Here's the drawing with two shaded views (mm, measured from the low corner). I have some questions. Round coordinates to 2 decimals unless told otherwise and drop trailing zeros. Loops run counter-clockwise (first coordinate to the right, second up) from the corner with the lowest first, then second, coordinate; pieces in that order, holes last. Notation, with made-up numbers: (8, -38) - (46, -38) arc R15 ccw to (46, -22) - close; hole circle Ø2 at (38, 21). An arc over 180 degrees is marked (long way). Answer as CSV lines item,"result".
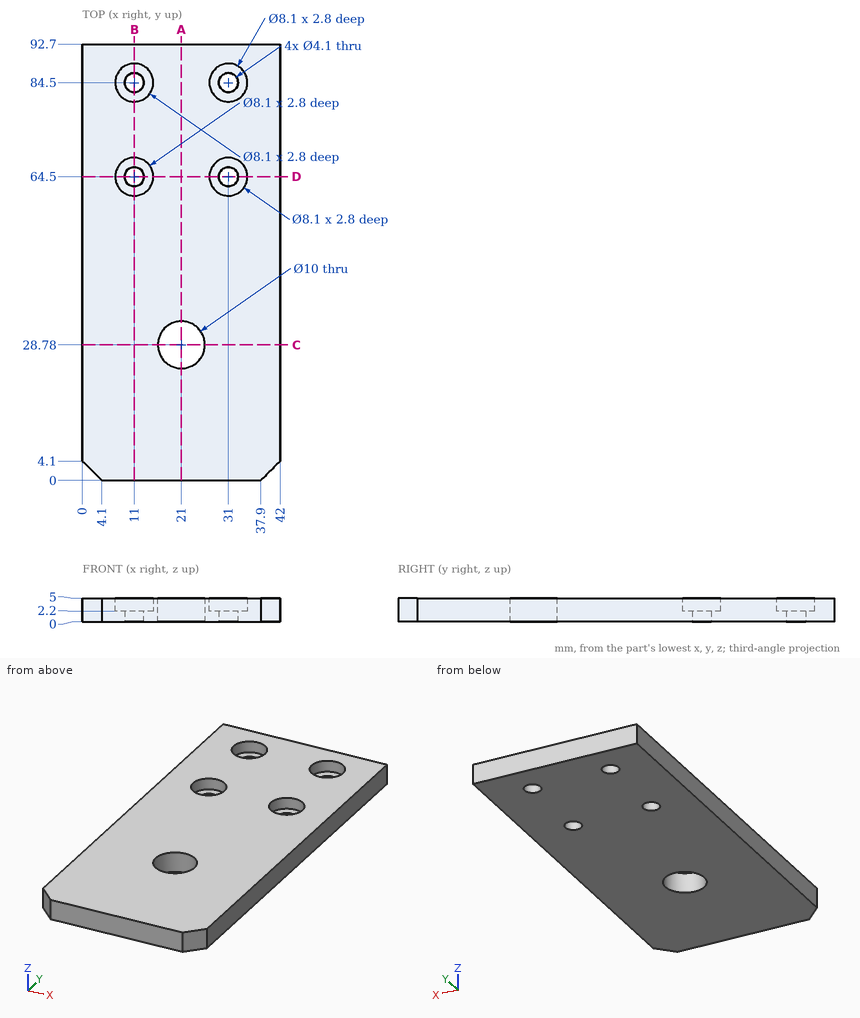
Q1. Imagine slicing it at C-C (y = 28.78). Write out the boundary of the cut face in (x, z), then the cut area to 3 significant figures.
Checks:
outline,"(0, 0) - (16, 0) - (16, 5) - (0, 5) - close; (26, 0) - (42, 0) - (42, 5) - (26, 5) - close"
area,"160 mm²"
Q2. Imagine slicing it at D-D (y = 64.5). Write out the boundary of the cut face in (x, z), then the cut area to 3 significant figures.
Checks:
outline,"(0, 0) - (8.95, 0) - (8.95, 2.2) - (6.95, 2.2) - (6.95, 5) - (0, 5) - close; (13.05, 0) - (28.95, 0) - (28.95, 2.2) - (26.95, 2.2) - (26.95, 5) - (15.05, 5) - (15.05, 2.2) - (13.05, 2.2) - close; (33.05, 0) - (42, 0) - (42, 5) - (35.05, 5) - (35.05, 2.2) - (33.05, 2.2) - close"
area,"147 mm²"
Q3. Imagine slicing it at B-B (x = 11). Write out the boundary of the cut face in (y, z), then the cut area to 3 significant figures.
Checks:
outline,"(0, 0) - (62.45, 0) - (62.45, 2.2) - (60.45, 2.2) - (60.45, 5) - (0, 5) - close; (66.55, 0) - (82.45, 0) - (82.45, 2.2) - (80.45, 2.2) - (80.45, 5) - (68.55, 5) - (68.55, 2.2) - (66.55, 2.2) - close; (86.55, 0) - (92.7, 0) - (92.7, 5) - (88.55, 5) - (88.55, 2.2) - (86.55, 2.2) - close"
area,"400 mm²"
Q4. I'm going to push a flat-ended pin straight in: pin 1 Ø4 at (x, y) = (10.5, 84) entering from +Z. Where does the tip first touch, or does it pass through?
Checks:
pin 1,"z = 2.2"
Q5. If I drill on line 1 along Y through (x, z) = (11, 3.7); line 2 along Y through (x, z) = (11, 1.7); line 3 along Y through (x, z) = (21, 3.75), over which ranges is the centre line in solid material (lowest first)? Write a range as [from, to].
Checks:
line 1,"[0, 60.45], [68.55, 80.45], [88.55, 92.7]"
line 2,"[0, 62.45], [66.55, 82.45], [86.55, 92.7]"
line 3,"[0, 23.78], [33.78, 92.7]"
Q6. Imagine slicing it at A-A (x = 21). Write out the boundary of the cut face in (y, z), then the cut area to 4 significant figures.
Checks:
outline,"(0, 0) - (23.78, 0) - (23.78, 5) - (0, 5) - close; (33.78, 0) - (92.7, 0) - (92.7, 5) - (33.78, 5) - close"
area,"413.5 mm²"
